Verification items for this drawing (mm, ordinates from the low corner). Give positions to 0.01 mm unless a question says otherwise; leave off trailing zeros. Loops run counter-clockwise (first coordinate to the right, second up) from the corner with the lowest first, then second, coordinate; pieces in that order, holes last. Notation, with made-up numbers: (52.5, 38) -> (67.5, 38) arc R19 ccw to (67.5, 46) -> close; hole circle Ø3 at (59.5, 88.5). An arc over 180 degrees is marked (long way). Write item = value, one per line.
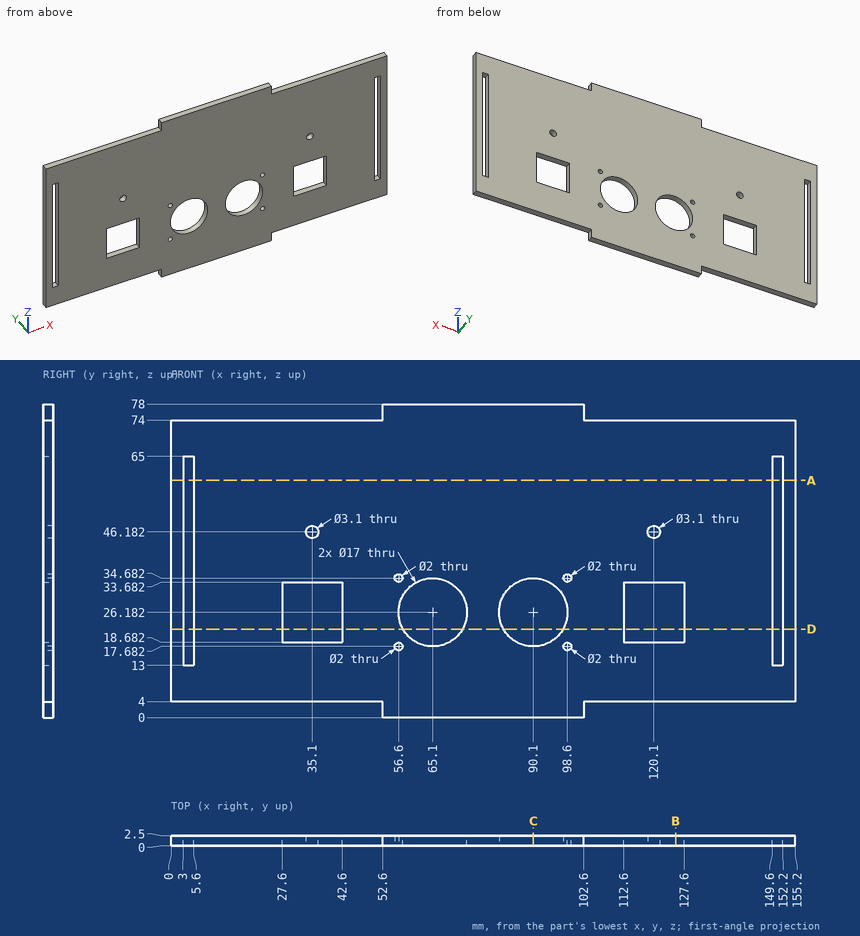
Item 1: Section check C-C, the plane x = 90.1. Record the cut outline in (y, z).
Answer:
outline = (0, 0) -> (2.5, 0) -> (2.5, 17.68) -> (0, 17.68) -> close; (0, 34.68) -> (2.5, 34.68) -> (2.5, 78) -> (0, 78) -> close
Item 2: Section check B-B, the plane x = 125.5. Record the cut outline in (y, z), plus the area to 4 significant figures.
Answer:
outline = (0, 4) -> (2.5, 4) -> (2.5, 18.68) -> (0, 18.68) -> close; (0, 33.68) -> (2.5, 33.68) -> (2.5, 74) -> (0, 74) -> close
area = 137.5 mm^2
Item 3: Thickness scan on L1, parallel to X at y = 1.9, z = 42; L2, parallel to X at y = 0.1, z = 46.5; L3, parallel to Z at x = 125, y = 0.8. Record the ranges inside material, lowest first. Write a range as [from, to].
Answer:
L1 = [0, 3], [5.6, 149.6], [152.2, 155.2]
L2 = [0, 3], [5.6, 33.58], [36.62, 118.58], [121.62, 149.6], [152.2, 155.2]
L3 = [4, 18.68], [33.68, 74]
Item 4: Gauge pin test, flat end, axial feed: pin 1 (1.2 mm diameter, centred on x = 15.5, y = 1, fed in from +Z). Record the tip position at first contact, or that the pin passes through.
Answer:
pin_1 = 74
Item 5: Section check D-D, the plane z = 22. Record the cut outline in (x, y).
Answer:
outline = (0, 0) -> (3, 0) -> (3, 2.5) -> (0, 2.5) -> close; (5.6, 0) -> (27.6, 0) -> (27.6, 2.5) -> (5.6, 2.5) -> close; (42.6, 0) -> (57.7, 0) -> (57.7, 2.5) -> (42.6, 2.5) -> close; (72.5, 0) -> (82.7, 0) -> (82.7, 2.5) -> (72.5, 2.5) -> close; (97.5, 0) -> (112.6, 0) -> (112.6, 2.5) -> (97.5, 2.5) -> close; (127.6, 0) -> (149.6, 0) -> (149.6, 2.5) -> (127.6, 2.5) -> close; (152.2, 0) -> (155.2, 0) -> (155.2, 2.5) -> (152.2, 2.5) -> close
Item 6: Section check A-A, the plane z = 59. Record the cut outline in (x, y).
Answer:
outline = (0, 0) -> (3, 0) -> (3, 2.5) -> (0, 2.5) -> close; (5.6, 0) -> (149.6, 0) -> (149.6, 2.5) -> (5.6, 2.5) -> close; (152.2, 0) -> (155.2, 0) -> (155.2, 2.5) -> (152.2, 2.5) -> close
